from build123d import *

# Parameters (mm, degrees)
CYLINDER215_R     = 3.75
CYLINDER215_DEPTH = 10
CYLINDER211_R     = 14.5
CYLINDER211_DEPTH = 29


with BuildPart() as cylinder215:
    # Cylinder215 → Cylinder215 (new body)
    with BuildSketch(Plane(origin=(0, -8, -36.5), x_dir=(1, 0, 0), z_dir=(0, -1, 0))):
        Circle(CYLINDER215_R)
    extrude(amount=CYLINDER215_DEPTH)


with BuildPart() as base011:
    # Cylinder211 → Cylinder211 (new body)
    with BuildSketch(Plane.XY.offset(-41.5)):
        Circle(CYLINDER211_R)
    extrude(amount=CYLINDER211_DEPTH)

    # Cut152: cut Cylinder215
    add(cylinder215.part, mode=Mode.SUBTRACT)


solid = base011.part
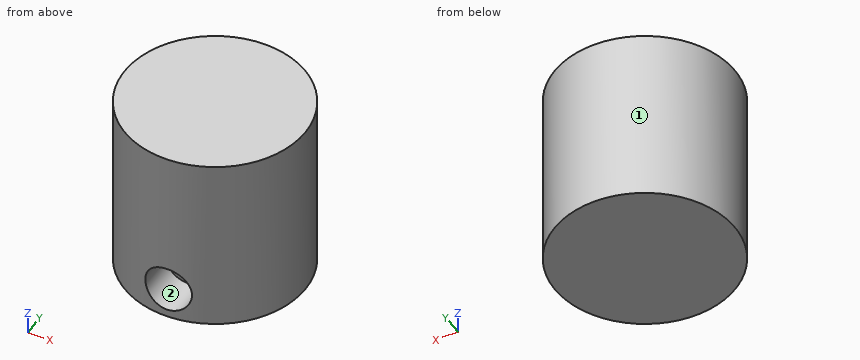
Source: CAD feature listing. Evaluate the final solid. Frame: model axes, mm. Face numbers are marked on the shaded views. A direction names the side the tool comes from. Give positions to 0.01 mm unless a question says otherwise; leave off trailing zeros. Write each loop counter-clockwise with the first axis right and the second up, starting at its lowest first coordinate (ties: lowest second). Pieces come first, ordered by that corner, then holes. Notation, with made-up numbers: M 55,-7.5 L 94,-7.5 A18 cw 94,13.5 Z; hole C 88,51.5 d4. An arc over 180 degrees is marked long. Answer as a JSON object with one key per item and string values.
Q1. Access query for the marked faces 1 and 2. Directions: +Z, -Z, +X, -X, +Y, -Y. A direction counts if a zero-diameter tool reaches every point of the face in a straight line with its end or side. Return the directions, or none.
Geometry check:
{"face 1": "+Z, -Z", "face 2": "-Y"}
Q2. Cut plane A-A, the plane x = 0. Return the cut outline in (y, z), then the cut area to 3 significant figures.
Geometry check:
{"outline": "M -14.5,-41.5 L 14.5,-41.5 L 14.5,-12.5 L -14.5,-12.5 L -14.5,-32.75 L -8,-32.75 L -8,-40.25 L -14.5,-40.25 Z", "area": "792 mm^2"}
Q3. Ray query, line 1 along Z through (x, y) = (0, -10); line 2 along X through (y, z) = (-10.75, -34.5); line 3 along X through (y, z) = (-9.5, -36.5). Return the intervals inside material, ascending.
Geometry check:
{"line 1": "z = -41.5 to -40.25, -32.75 to -12.5", "line 2": "x = -9.73 to -3.17, 3.17 to 9.73", "line 3": "x = -10.95 to -3.75, 3.75 to 10.95"}
Q4. Cut plane D-D, the plane x = 3.25. Return the cut outline in (y, z).
Geometry check:
{"outline": "M -14.13,-41.5 L 14.13,-41.5 L 14.13,-12.5 L -14.13,-12.5 L -14.13,-34.63 L -8,-34.63 L -8,-38.37 L -14.13,-38.37 Z"}
Q5. Cut plane B-B, the plane z = -27.5. Return the cut outline in (x, y).
Geometry check:
{"outline": "C 0,0 d29"}
Q6. Contact query for flat-ended pins moving along their axis: P1, Ø5, axis at x = 8, z = -25.5, coming from the -Y side; P2, Ø4.5, axis at x = 0, z = -36.5, coming from the -Y side; P3, Ø4, axis at y = -5.5, z = -32, coming from the +X side. Output: stop coordinate, or through.
Geometry check:
{"P1": "stops at y = -13.42", "P2": "stops at y = -8", "P3": "stops at x = 14.07"}
Q7. Cut plane C-C, the plane y = 5. Return the cut outline in (x, z).
Geometry check:
{"outline": "M -13.61,-41.5 L 13.61,-41.5 L 13.61,-12.5 L -13.61,-12.5 Z"}
